```python
from build123d import *

# Parameters (mm, degrees)
CROQUIS1_W              = 24
CROQUIS1_H              = 144
SALIENTE_EXTRUIR1_DEPTH = 20
CORTAR_EXTRUIR2_DEPTH   = 148.349923651
CROQUIS7_W              = 24
CROQUIS7_H              = 40.261393694
CROQUIS4_W              = 24
CROQUIS4_H              = 90


with BuildPart() as part:
    # Croquis1 → Saliente-Extruir1 (new body)
    with BuildSketch(Plane(origin=(0, 0, 0), x_dir=(1, 0, 0), z_dir=(0, 1, 0))):
        with Locations((12, 72)):
            Rectangle(CROQUIS1_W, CROQUIS1_H)
    extrude(amount=SALIENTE_EXTRUIR1_DEPTH)

    # Croquis3 → Cortar-Extruir2 (cut, through all)
    with BuildSketch(Plane(origin=(24, 0, 0), x_dir=(0, 0, -1), z_dir=(1, 0, 0))):
        Polygon((144, 20), (0, 0), (0, 20), align=None)
    extrude(amount=-CORTAR_EXTRUIR2_DEPTH, mode=Mode.SUBTRACT)

    # Croquis7 → Cortar-Revolución5 (revolve, cut)
    with BuildSketch(Plane.XZ):
        with Locations((12, -164.130696847)):
            Rectangle(CROQUIS7_W, CROQUIS7_H)
    revolve(axis=Axis((0, 0, 0), (1, 0, 0)), mode=Mode.SUBTRACT)

    # Croquis4 → Cortar-Revolución3 (revolve, cut)
    with BuildSketch(Plane.XZ):
        with Locations((12, -45)):
            Rectangle(CROQUIS4_W, CROQUIS4_H)
    revolve(axis=Axis((24, 0, 0), (-1, 0, 0)), mode=Mode.SUBTRACT)


solid = part.part
```
Geometry: final body of the model. Coordinates: model frame, mm. Coordinates: 2 decimals unless noted, no trailing zeros. Order: outer loops, then holes, each group sorted by start corner. A loop starts at its lowest first (then second) coordinate and runs counter-clockwise, first axis right, second up. Notation, with made-up numbers: M 14.25,-3.75 L 22.25,-3.75 A4 ccw 22.25,0.25 Z; hole C -33.5,-39 d5. An arc over 180 degrees is marked long. Answer in a Markdown table with one row per item. Add a question column.
Q1. Section query B-B on x = 9. Return the cut outline in (y, z), and give its area (3 significant figures).
Q2. Line query: L1, parallel to Y at x = 22.75, z = -111; L2, parallel to Z at x = 18.75, y = 4.25; L3, parallel to Z at x = 8, y = 9. Output: solid intervals per line, ascending.
Q3. Section query A-A on z = -113. Return the cut outline in (x, y).
Q4. Contact query for flat-ended pins moving along their axis: P1, Ø12, axis at x = 21, z = -106.5, coming from the +Y side (3 decimals); P2, Ø12, axis at x = 15, z = -127.5, coming from the +Y side; P3, Ø5, axis at x = 5.5, z = -108, coming from the +Y side. Output: stop coordinate, or through.
Completed:
| question | item | result |
|---|---|---|
| 1 | outline | M 0,-144 A144 ccw 19.81,-142.63 L 12.38,-89.14 A90 cw 0,-90 Z |
| 1 | area | 872 mm2 |
| 2 | L1 | y = 0 to 15.42 |
| 2 | L2 | z = -143.94 to -89.9 |
| 2 | L3 | z = -143.72 to -89.55 |
| 3 | outline | M 0,0 L 24,0 L 24,15.69 L 0,15.69 Z |
| 4 | P1 | stops at y = 15.625 |
| 4 | P2 | stops at y = 18.54 |
| 4 | P3 | stops at y = 15.35 |
